```python
from build123d import *

# Parameters (mm, degrees)
F0_R            = 14
F0_W            = 12.5
F0_H            = 12.5
F1_DEPTH        = 130
F2_R            = 2.5
F4_DEPTH        = 25
F3_R            = 2.5
F5_DEPTH        = 25
F9_DEPTH        = 1
F9_COPIES_COUNT = 3
F9_COPIES_ANGLE = 180
F12_R           = 5
F13_DEPTH       = 1


# Not quite as in the source:
# - a pattern or mirror of a feature is missing from the dataset's text; its kind, count and spacing are read off the source's solid


with BuildPart() as f1:
    # F0 (on Top) → F1 (new body)
    with BuildSketch(Plane.XY):
        Circle(F0_R)
        Rectangle(F0_W, F0_H, mode=Mode.SUBTRACT)
    extrude(amount=F1_DEPTH)

    # F2 (on face) → F4 (cut, symmetric)
    with BuildSketch(Plane.XZ.offset(-6.25)):
        with Locations((0, 10)):
            Circle(F2_R)
        with Locations((0, 120)):
            Circle(F2_R)
    extrude(amount=F4_DEPTH, both=True, mode=Mode.SUBTRACT)

    # F3 (on face) → F5 (cut, symmetric)
    with BuildSketch(Plane.YZ.offset(-6.25)):
        with BuildLine():
            ThreePointArc((2.5, 120), (1.767766953, 121.767766953), (0, 122.5))
            ThreePointArc((0, 122.5), (-1.767766953, 118.232233047), (2.5, 120))
        make_face()
        with Locations((0, 10)):
            Circle(F3_R)
    extrude(amount=F5_DEPTH, both=True, mode=Mode.SUBTRACT)

    # F8 (on line) → F9 (cut)
    with BuildSketch(Plane(origin=(14, 0, 0), x_dir=(0, -1, 0), z_dir=(-1, 0, 0))):
        with BuildLine():
            ThreePointArc((5, 120), (3.5355339059, 123.5355339059), (0, 125))
            Line((0, 125), (0, 115))
            ThreePointArc((0, 115), (3.5355339059, 116.4644660941), (5, 120))
        make_face()
        with BuildLine():
            ThreePointArc((5, 10), (3.5355339059, 13.5355339059), (0, 15))
            Line((0, 15), (0, 5))
            ThreePointArc((0, 5), (3.5355339059, 6.4644660941), (5, 10))
        make_face()
        with BuildLine():
            Line((0, 5), (0, 15))
            ThreePointArc((0, 15), (-5, 10), (0, 5))
        make_face()
        with BuildLine():
            Line((0, 115), (0, 125))
            ThreePointArc((0, 125), (-5, 120), (0, 115))
        make_face()
    f9 = extrude(amount=F9_DEPTH, mode=Mode.SUBTRACT)

    # F9_copies: F9 ×3 about axis
    f9_copies_axis = Axis((0, 0, 0), (0, 0, 1))
    for i in range(1, F9_COPIES_COUNT):
        add(f9.rotate(f9_copies_axis, i * F9_COPIES_ANGLE / (F9_COPIES_COUNT - 1)), mode=Mode.SUBTRACT)

    # F12 (on line) → F13 (cut)
    with BuildSketch(Plane(origin=(0, -14, 0), x_dir=(-1, 0, 0), z_dir=(0, 1, 0))):
        with BuildLine():
            ThreePointArc((0, 125), (-3.5355339059, 116.4644660941), (5, 120))
            ThreePointArc((5, 120), (3.5355339059, 123.5355339059), (0, 125))
        make_face()
        with Locations((0, 10)):
            Circle(F12_R)
    extrude(amount=F13_DEPTH, mode=Mode.SUBTRACT)


solid = f1.part
```
Input: part model. Units: mm. Frame: model coordinates. A direction names the side the tool comes from. Round coordinates to 2 decimals unless told otherwise and drop trailing zeros. Loops run counter-clockwise (first coordinate to the right, second up) from the corner with the lowest first, then second, coordinate; pieces in that order, holes last. Notation, with made-up numbers: (39, 31.25) -> (50, 31.25) arc R21 ccw to (50, 59.25) -> close; hole circle Ø8 at (54.5, 26). An arc over 180 degrees is marked (long way). Use one line per item in the form item = value. Start each with the question number.
Item 1: Material intervals for L1, parallel to Z at x = 0.25, y = 10; L2, parallel to Z at x = -11.25, y = -1.5; L3, parallel to Y at x = -0.75, z = 114, sorted ascending. Write a range as from..to.
Item 2: Section query C-C on z = 17. Return the cut outline in (x, y).
Item 3: Section query D-D on y = 8. Return the cut outline in (x, z).
Item 4: Section query B-B on x = -9. Return the cut outline in (y, z).
Item 5: Set-up query: faces 1 (the face through (-6.25, 0, 64)), 2 (the face through (-13, 2, 8)), 3 (the face through (-2, -13, 8)), 4 (the face through (13, -2, 118)). Return all of +Z, -Z, +X, -X, +Y, -Y with unobstructed straight access to the full face (end or side cutting, diameter ignored); none if empty.
Item 6: Contact query for flat-ended pins moving along their axis: pin 1 Ø11 at (x, z) = (-1, 10) entering from -Y; pin 2 Ø6 at (y, z) = (0, 10) entering from +X; pin 3 Ø6 at (x, z) = (-11, 23.5) entering from -Y; pin 4 Ø3 at (y, z) = (0.5, 121.5) entering from -X. Output: stop coordinate, or through.
Item 7: Mould query, pull axis Z, two halves, no side actions, for faces 5 (the face through (-6.4, 0.2, 130)), 6 (the face through (6.25, 0, 64)), 7 (the face through (-0.54, -9.58, 7.56)). Classes: pulls with the +Z half, pulls with the -Z half, needs draft (parallel to the pull), parting line crosses it, or undercut.
Item 8: Section query A-A on y = -3.75. Return the cut outline in (x, z).
Ans:
q1.L1 = 0..7.51, 12.49..117.51, 122.49..130
q1.L2 = 0..8, 12..118, 122..130
q1.L3 = -13.98..-6.25, 6.25..13.98
q2.outline = circle Ø28 at (0, 0); hole (-6.25, -6.25) -> (6.25, -6.25) -> (6.25, 6.25) -> (-6.25, 6.25) -> close
q3.outline = (-11.49, 0) -> (11.49, 0) -> (11.49, 130) -> (-11.49, 130) -> close; hole circle Ø5 at (0, 10); hole circle Ø5 at (0, 120)
q4.outline = (-10.72, 0) -> (10.72, 0) -> (10.72, 130) -> (-10.72, 130) -> close; hole circle Ø5 at (0, 10); hole circle Ø5 at (0, 120)
q5.face_1 = +Z, -Z
q5.face_2 = -X
q5.face_3 = -Y
q5.face_4 = +X
q6.pin_1 = -14
q6.pin_2 = 13
q6.pin_3 = -11.49
q6.pin_4 = -13
q7.face_5 = pulls with the +Z half
q7.face_6 = needs draft
q7.face_7 = undercut
q8.outline = (-13.49, 0) -> (-6.25, 0) -> (-6.25, 130) -> (-13.49, 130) -> (-13.49, 123.31) -> (-13, 123.31) -> (-13, 116.69) -> (-13.49, 116.69) -> (-13.49, 13.31) -> (-13, 13.31) -> (-13, 6.69) -> (-13.49, 6.69) -> close; (6.25, 0) -> (13.49, 0) -> (13.49, 6.69) -> (13, 6.69) -> (13, 13.31) -> (13.49, 13.31) -> (13.49, 116.69) -> (13, 116.69) -> (13, 123.31) -> (13.49, 123.31) -> (13.49, 130) -> (6.25, 130) -> close
